Geometry check sheet. Reference: the model listing, model coordinates, mm. Round coordinates to 2 decimals unless told otherwise and drop trailing zeros. Write each loop counter-clockwise with the first axis right and the second up, starting at its lowest first coordinate (ties: lowest second). Pieces come first, ordered by that corner, then holes. Notation, with made-up numbers: M -1.5,-16.5 L 14.5,-16.5 A15 ccw 14.5,-0.5 Z; hole C 16,26 d11. An arc over 180 degrees is marked long. Use a Markdown table: item, result.
```python
from build123d import *

# Parameters (mm, degrees)
ESQUISSE1_W         = 17.873
ESQUISSE1_H         = 13.873
BOARD_OUTLINE_DEPTH = 1.6
ESQUISSE2_R         = 1.5
NPTH_DEPTH          = 2.6
ESQUISSE3_R         = 0.51
PTH_DEPTH           = 2.6
CHANFREIN1_SIZE     = 3


with BuildPart() as part:
    # Esquisse1 → Board_Outline (new body)
    with BuildSketch(Plane.XY):
        with Locations((8.4285, 5.1585)):
            Rectangle(ESQUISSE1_W, ESQUISSE1_H)
    extrude(amount=BOARD_OUTLINE_DEPTH)

    # Esquisse2 → NPTH (cut, through all)
    with BuildSketch(Plane.XY):
        with Locations((12.7, 0.5)):
            Circle(ESQUISSE2_R)
    extrude(amount=NPTH_DEPTH, mode=Mode.SUBTRACT)

    # Esquisse3 → PTH (cut, through all)
    with BuildSketch(Plane.XY):
        with Locations((3.81, 2.54)):
            Circle(ESQUISSE3_R)
        with Locations((3.81, 5.08)):
            Circle(ESQUISSE3_R)
        with Locations((3.81, 7.62)):
            Circle(ESQUISSE3_R)
    extrude(amount=PTH_DEPTH, mode=Mode.SUBTRACT)

    # Chanfrein1
    chanfrein1_edges = [part.edges().sort_by_distance(p)[0] for p in [
        (-0.508, -1.778, 0.8),
        (-0.508, 12.095, 0.8),
        (17.365, 12.095, 0.8),
        (17.365, -1.778, 0.8),
    ]]
    chamfer(chanfrein1_edges, length=CHANFREIN1_SIZE)


solid = part.part
```
Item 1: Go/stop test with a flat-tipped pin: pin 1 (0.9 mm diameter, centred on x = 3.81, y = 5.08, fed in from -Z). Record where the tip stops, or that it passes through.
Outcome:
| item | result |
|---|---|
| pin 1 | passes through |
Item 2: Cross-section at B-B, the plane y = 7.62. Record the cut outline in (x, z) (3 decimals).
Outcome:
| item | result |
|---|---|
| outline | M -0.508,0 L 3.3,0 L 3.3,1.6 L -0.508,1.6 Z; M 4.32,0 L 17.365,0 L 17.365,1.6 L 4.32,1.6 Z |
Item 3: Cross-section at A-A, the plane x = 12.7. Record the cut outline in (y, z) (3 decimals).
Outcome:
| item | result |
|---|---|
| outline | M -1.778,0 L -1,0 L -1,1.6 L -1.778,1.6 Z; M 2,0 L 12.095,0 L 12.095,1.6 L 2,1.6 Z |
Item 4: Material ranges on line 1 along Y through (x, z) = (3.81, 0.4) (3 decimals); line 2 along X through (y, z) = (5.08, 1.3) (3 decimals); line 3 along Y through (x, z) = (12.7, 1.15) (3 decimals), recorded low to high. Write a range as from..to.
Outcome:
| item | result |
|---|---|
| line 1 | y = -1.778..2.03, 3.05..4.57, 5.59..7.11, 8.13..12.095 |
| line 2 | x = -0.508..3.3, 4.32..17.365 |
| line 3 | y = -1.778..-1, 2..12.095 |
Item 5: Cross-section at C-C, the plane x = 3.81. Record the cut outline in (y, z) (3 decimals), and give its area (3 significant figures).
Outcome:
| item | result |
|---|---|
| outline | M -1.778,0 L 2.03,0 L 2.03,1.6 L -1.778,1.6 Z; M 3.05,0 L 4.57,0 L 4.57,1.6 L 3.05,1.6 Z; M 5.59,0 L 7.11,0 L 7.11,1.6 L 5.59,1.6 Z; M 8.13,0 L 12.095,0 L 12.095,1.6 L 8.13,1.6 Z |
| area | 17.3 mm2 |
Item 6: Mould release check, pull along X, two halves, no side actions. Record for faces 1 (the face through (3.744, 5.586, 0.789)), 2 (the face through (15.886, -0.257, 0.789)), 3 (the face through (8, -1.778, 1)): +X half, -X half, draft (parallel to the pull), parting line (faces both ways), or undercut.
Outcome:
| item | result |
|---|---|
| face 1 | undercut |
| face 2 | +X half |
| face 3 | draft |
Item 7: Cross-section at D-D, the plane z = 1.3. Record the cut outline in (x, y) (3 decimals).
Outcome:
| item | result |
|---|---|
| outline | M -0.508,1.222 L 2.492,-1.778 L 14.365,-1.778 L 17.365,1.222 L 17.365,9.095 L 14.365,12.095 L 2.492,12.095 L -0.508,9.095 Z; hole C 3.81,2.54 d1.02; hole C 3.81,5.08 d1.02; hole C 3.81,7.62 d1.02; hole C 12.7,0.5 d3 |
